Design review of the part shown in the three views and the two pictorial views. Dimensions are in mm from the part's minimum x, y and z. Coordinates: 2 decimals unless noted, no trailing zeros. Write item = value, one per line. Start each with the question number.
1) Insertion check: pin 1 Ø16 at (x, y) = (46.72, 103.28) entering from +Z; pin 2 Ø2 at (y, z) = (80, 3) entering from -X. Each pin has a flat end and moves straight along its axis. Give the tip position at first contact, or say it passes through.
2) Wall thickness on probe 1 along X at (y, z) = (49.5, 2.6) (1 decimal); probe 2 along Y at (x, z) = (75, 1.45) (1 decimal); probe 3 along X at (y, z) = (41, 3.85) (1 decimal): over which ranges is each line inside the solid? List them lowest first. Write a range as [from, to].
3) Consider section A-A on y = 75. State how many separate pieces and enclosed holes the cut face has, and give its area (3 significant figures).
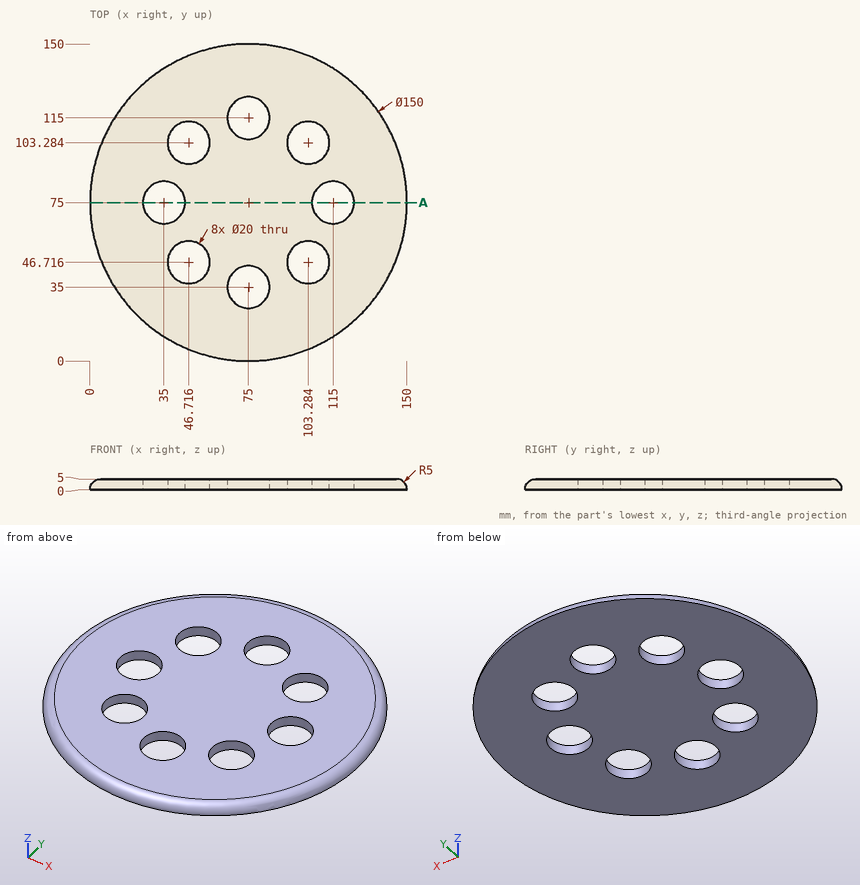
Answer sheet:
q1.pin_1 = through
q1.pin_2 = 0.58
q2.probe_1 = [5.2, 37.1], [56.3, 93.7], [112.9, 144.8]
q2.probe_2 = [0.2, 25], [45, 105], [125, 149.8]
q2.probe_3 = [10.2, 38.5], [54.9, 67], [83, 95.1], [111.5, 139.8]
q3.separate_pieces = 3
q3.enclosed_holes = 0
q3.area = 539 mm2
